```python
from build123d import *

# Parameters (mm, degrees)
SKETCH_1_R             = 3
EXTRUDE_1_DEPTH        = 2
SKETCH_2_W             = 53.96
SKETCH_2_H             = 15
SKETCH_2_R             = 1.6
SKETCH_2_R_2           = 1
EXTRUDE_2_DEPTH        = 2
PATTERN_LINEAR_1_COUNT = 2
PATTERN_LINEAR_1_PITCH = 13
FILLET_1_R             = 1
EXTRUDE_START          = -16
SKETCH_4_R             = 3
EXTRUDE_3_DEPTH        = 16
SKETCH_5_W             = 71.597299473
SKETCH_5_H             = 10
CUT_EXTRUDE_1_DEPTH    = 15
SKETCH_6_R             = 5
CUT_EXTRUDE_2_DEPTH    = 3
CUT_EXTRUDE_START      = -3
SKETCH_7_R             = 5
CUT_EXTRUDE_3_DEPTH    = 3
FILLET_2_R             = 10
SKETCH_8_W             = 2
SKETCH_8_H             = 0.095117033
EXTRUDE_5_DEPTH        = 0.002
CUT_EXTRUDE_4_DEPTH    = 16
FILLET_3_R             = 3
CUT_EXTRUDE_5_REACH    = 63.416
SKETCH_11_W            = 36.223911337
SKETCH_11_H            = 10
SKETCH_14_W            = 10
SKETCH_14_H            = 20
CUT_EXTRUDE_6_DEPTH    = 8
HOLE_WIZARD_M3_1_D     = 2.5
HOLE_WIZARD_M3_1_DEPTH = 7.5
HOLE_WIZARD_M3_1_TIP   = 0.751075774


with BuildPart() as part:
    # 草图1 → 凸台-拉伸1 (new body)
    with BuildSketch(Plane.XY):
        with BuildLine():
            Line((-31.667580782, -19.712759913), (-15.214545893, -22.177554229))
            Line((-15.214545893, -22.177554229), (-14.362700527, -22.30516738))
            Line((-14.362700527, -22.30516738), (-14.362700527, -23.166518437))
            Line((-14.362700527, -23.166518437), (-14.362700527, -25.01516738))
            Line((-14.362700527, -25.01516738), (39.597299473, -25.01516738))
            Line((39.597299473, -25.01516738), (39.597299473, -20.01516738))
            Line((39.597299473, -20.01516738), (-6.399297664, -20.01516738))
            Line((-6.399297664, -20.01516738), (-6.399297664, 14.684969608))
            ThreePointArc((-6.399297664, 14.684969608), (-6.397869517, 15.219044335), (-6.427963434, 15.752272438))
            ThreePointArc((-6.427963434, 15.752272438), (-6.435285609, 15.800138476), (-6.441446817, 15.848167752))
            ThreePointArc((-6.441446817, 15.848167752), (-13.325191112, 23.766199394), (-23.057324529, 19.846156059))
            Line((-23.057324529, 19.846156059), (-38.645044316, -4.254376507))
            ThreePointArc((-38.645044316, -4.254376507), (-39.369264732, -13.885171984), (-31.667580782, -19.712759913))
        make_face()
        with Locations((-30.439815615, -11.004528038)):
            Circle(SKETCH_1_R, mode=Mode.SUBTRACT)
        with Locations((-15.440178747, 14.976184715)):
            Circle(SKETCH_1_R, mode=Mode.SUBTRACT)
    extrude_1 = extrude(amount=EXTRUDE_1_DEPTH)

    # 草图2 → 凸台-拉伸2 (add)
    with BuildSketch(Plane.XZ.offset(25.01516738)):
        with Locations((12.617299473, -5.5)):
            Rectangle(SKETCH_2_W, SKETCH_2_H)
        with Locations(Location((26.637299473, -5.5, 0), (0, 0, 270))):
            Circle(SKETCH_2_R, mode=Mode.SUBTRACT)
        with Locations(Location((-9.362700527, -5.5, 0), (0, 0, 270))):
            Circle(SKETCH_2_R, mode=Mode.SUBTRACT)
        with Locations(Location((-3.141180602, -5.5, 0), (0, 0, 270))):
            Circle(SKETCH_2_R_2, mode=Mode.SUBTRACT)
        with Locations(Location((20.358819398, -5.5, 0), (0, 0, 270))):
            Circle(SKETCH_2_R_2, mode=Mode.SUBTRACT)
        with BuildLine():
            Line((3.367759388, -1.25), (-1.491180602, -1.25))
            Line((-1.491180602, -1.25), (-1.491180602, -9.75))
            Line((-1.491180602, -9.75), (3.367759388, -9.75))
            ThreePointArc((3.367759388, -9.75), (6.858819398, -11), (10.349879409, -9.75))
            Line((10.349879409, -9.75), (18.708819398, -9.75))
            Line((18.708819398, -9.75), (18.708819398, -1.25))
            Line((18.708819398, -1.25), (10.349879409, -1.25))
            ThreePointArc((10.349879409, -1.25), (6.858819398, 0), (3.367759388, -1.25))
        make_face(mode=Mode.SUBTRACT)
    extrude(amount=-EXTRUDE_2_DEPTH)

    # 阵列(线性)1: 凸台-拉伸1 ×2
    with Locations(*[(0, 0, -i * PATTERN_LINEAR_1_PITCH) for i in range(1, PATTERN_LINEAR_1_COUNT)]):
        add(extrude_1)

    # 圆角1
    fillet_1_edges = [part.edges().sort_by_distance(p)[0] for p in [
        (-14.362700527, -22.30516738, -12),
    ]]
    fillet(fillet_1_edges, radius=FILLET_1_R - 0.0004)  # a hair under: the kernel refuses the full size

    # 草图4 → 凸台-拉伸3 (add)
    with BuildSketch(Plane.XY.offset(2).offset(EXTRUDE_START)):
        Polygon((-20.359667451, 24.017065798), (-48.838793814, -20.01516738), (-6.299297664, -20.01516738), (-6.299297664, 24.017065798), align=None)
        with Locations((-15.440178747, 14.976184715)):
            Circle(SKETCH_4_R, mode=Mode.SUBTRACT)
        with Locations((-30.439815615, -11.004528038)):
            Circle(SKETCH_4_R, mode=Mode.SUBTRACT)
    extrude(amount=EXTRUDE_3_DEPTH)

    # 草图5 → 切除-拉伸1 (cut)
    with BuildSketch(Plane.XY.offset(2)):
        with Locations((3.798649736, -25.01516738)):
            Rectangle(SKETCH_5_W, SKETCH_5_H)
    extrude(amount=-CUT_EXTRUDE_1_DEPTH, mode=Mode.SUBTRACT)

    # 草图6 → 切除-拉伸2 (cut)
    with BuildSketch(Plane.XY.offset(2)):
        with Locations((-30.439815615, -11.004528038)):
            Circle(SKETCH_6_R)
    extrude(amount=-CUT_EXTRUDE_2_DEPTH, mode=Mode.SUBTRACT)

    # 草图7 → 切除-拉伸3 (cut)
    with BuildSketch(Plane(origin=(0, 0, -14), x_dir=(-1, 0, 0), z_dir=(0, 0, -1)).offset(CUT_EXTRUDE_START)):
        with Locations(Location((30.439815615, -11.004528038, 0), (0, 0, 180))):
            Circle(SKETCH_7_R)
    extrude(amount=CUT_EXTRUDE_3_DEPTH, mode=Mode.SUBTRACT)

    # 圆角2
    fillet_2_edges = [part.edges().sort_by_distance(p)[0] for p in [
        (-48.838793814, -20.01516738, -6),
    ]]
    fillet(fillet_2_edges, radius=FILLET_2_R)

    # 草图8 → 凸台-拉伸5 (add)
    with BuildSketch(Plane(origin=(-25.306928561, 16.367991454, 0), x_dir=(0, 0, 1), z_dir=(-0.8396772833764469, 0.5430856836462826, 0))):
        with Locations((-12, 4.189822066)):
            Rectangle(SKETCH_8_W, SKETCH_8_H)
        with Locations((1, 4.189822066)):
            Rectangle(SKETCH_8_W, SKETCH_8_H)
    extrude(amount=EXTRUDE_5_DEPTH)

    # 草图9 → 切除-拉伸4 (cut)
    with BuildSketch(Plane.XY.offset(2)):
        Polygon((-23.00566783, 19.926023671), (-23.057324529, 19.846156059), (-23.897001813, 20.389241743), (-23.845345113, 20.469109355), align=None)
    extrude(amount=-CUT_EXTRUDE_4_DEPTH, mode=Mode.SUBTRACT)

    # 圆角3
    fillet_3_edges = [part.edges().sort_by_distance(p)[0] for p in [
        (-20.359667451, 24.017065798, -6),
        (-6.299297664, 24.017065798, -6),
    ]]
    fillet(fillet_3_edges, radius=FILLET_3_R)

    # 切除-拉伸5: up to this face of the body (flat: up to its plane)
    cut_extrude_5_end = Plane(part.part.faces().sort_by_distance((-18.380481786, -20.01516738, -6))[0])
    # 草图11 → 切除-拉伸5 (cut, up to the picked face)
    with BuildSketch(Plane(origin=(0, 24.017065798, 0), x_dir=(1, 0, 0), z_dir=(0, 1, 0)), mode=Mode.PRIVATE) as cut_extrude_5_sk1:
        with Locations((-32.411253333, 6)):
            Rectangle(SKETCH_11_W, SKETCH_11_H)
    cut_extrude_5_tool1 = split(extrude(cut_extrude_5_sk1.sketch, amount=-CUT_EXTRUDE_5_REACH, mode=Mode.PRIVATE), bisect_by=cut_extrude_5_end, keep=Keep.BOTH, mode=Mode.PRIVATE)
    add(cut_extrude_5_tool1.solids().sort_by(Axis((-32.411253, 24.017066, -6), (0, -1, 0)))[0], mode=Mode.SUBTRACT)

    # 草图14 → 切除-拉伸6 (cut)
    with BuildSketch(Plane.ZY.offset(14.299297664)):
        with Locations((-6, 14.017065798)):
            Rectangle(SKETCH_14_W, SKETCH_14_H)
    extrude(amount=-CUT_EXTRUDE_6_DEPTH, mode=Mode.SUBTRACT)

    # M3 螺纹孔1
    with Locations(Plane(origin=(-6.299297664, 0, 0), x_dir=(0, 0, -1), z_dir=(1, 0, 0))):
        with Locations((2, -0.01516738), (10, -0.01516738), (2, -16.01516738), (10, -16.01516738)):
            Hole(HOLE_WIZARD_M3_1_D / 2, depth=HOLE_WIZARD_M3_1_DEPTH)
            with Locations((0, 0, -(HOLE_WIZARD_M3_1_DEPTH + HOLE_WIZARD_M3_1_TIP / 2))):  # 118° drill point
                Cone(0, HOLE_WIZARD_M3_1_D / 2, HOLE_WIZARD_M3_1_TIP, mode=Mode.SUBTRACT)


solid = part.part
```
Verification items for the finished model (mm, model axes). A direction names the side the tool comes from. Give positions to 0.01 mm unless a question says otherwise; leave off trailing zeros. Order: outer loops, then holes, each group sorted by start corner. A loop starts at its lowest first (then second) coordinate and runs counter-clockwise, first axis right, second up. Notation, with made-up numbers: (85.5, 55) -> (89.5, 55) arc R28 cw to (89.5, 84) -> close; hole circle Ø5 at (-28.5, -25.5). An arc over 180 degrees is marked (long way). One line per item, written item: value.
(1) Sectioned sample at A-A on x = -31. Record the cut outline in (y, z).
Final values:
outline: (-20, -14) -> (-15.97, -14) -> (-15.97, -11) -> (-20, -11) -> close; (-20, -1) -> (-15.97, -1) -> (-15.97, 2) -> (-20, 2) -> close; (-6.04, -14) -> (7.57, -14) -> (7.57, -11) -> (-6.04, -11) -> close; (-6.04, -1) -> (7.57, -1) -> (7.57, 2) -> (-6.04, 2) -> close
(2) Scan lines: line 1 along Y through (x, z) = (-8.5, -2); line 2 along Z through (x, y) = (-30.5, 0.5); line 3 along Y through (x, z) = (-13, -9). Record each from-to range of solid material in increasing order. Write a range as [from, to].
Final values:
line 1: [-20.02, -17.27], [-14.77, -1.27], [1.23, 4.02]
line 2: [-14, -11], [-1, 2]
line 3: [-20.02, -16.77], [-15.27, -0.77], [0.73, 4.02]
(3) Sectioned sample at D-D on y = 2.5. Record the cut outline in (x, z).
Final values:
outline: (-34.28, -14) -> (-6.3, -14) -> (-6.3, 2) -> (-34.28, 2) -> (-34.28, -1) -> (-14.3, -1) -> (-14.3, -11) -> (-34.28, -11) -> close
(4) Gauge pin test, flat ends, axial feed: pin 1 (5 mm diameter, centred on y = 8.5, z = -1, fed in from -X); pin 2 (4 mm diameter, centred on y = -0.02, z = -10, fed in from -X); pin 3 (6.5 mm diameter, centred on x = -10, z = -6, fed in from +Y). Record the tip position at first contact, or that the pin passes through.
Final values:
pin 1: x = -32.01
pin 2: x = -37.03
pin 3: y = 4.02
(5) Draft check along X on faces 5 (the face through (-14, 24.017, -13)), 6 (the face through (-15.83, 17.95, 0.48)), 7 (the face through (-7.2, 23.16, -12.48)). Enter one of: pulls with the +X half, pulls with the -X half, needs draft (parallel to the pull), parting line crosses it, or undercut.
Final values:
face 5: needs draft
face 6: undercut
face 7: pulls with the +X half
(6) Sectioned sample at B-B on x = -36. Record the cut outline in (y, z).
Final values:
outline: (-18.34, -14) -> (-0.16, -14) -> (-0.16, -11) -> (-18.34, -11) -> close; (-18.34, -1) -> (-0.16, -1) -> (-0.16, 2) -> (-18.34, 2) -> close
(7) Sectioned sample at C-C on z = -5.25. Record the cut outline in (x, y), then the cut area to 3 significant figures.
Final values:
outline: (-14.3, -20.02) -> (-6.3, -20.02) -> (-6.3, 4.02) -> (-14.3, 4.02) -> close
area: 192 mm^2
(8) Tool access check on faces 1 (the face through (-24, 2, -1)), 2 (the face through (-34.13, -14.38, -12.48)), 3 (the face through (-10.1, 0.04, -11.25)), 4 (the face through (-10, 4.017, -6)). Record the directions out of +Z, -Z, +X, -X, +Y, -Y that give a thin tool (end or side, any length) a straight path to the whole face; none if there is none.
Final values:
face 1: -X, +Y
face 2: +Z, -Z
face 3: +X
face 4: +X, -X, +Y
